Check sheet for the modelled part. Datum: model origin and axes. Units: mm. A direction names the side the tool comes from. Give positions to 0.01 mm unless a question says otherwise; leave off trailing zeros. Loops run counter-clockwise (first coordinate to the right, second up) from the corner with the lowest first, then second, coordinate; pieces in that order, holes last. Notation, with made-up numbers: (-10, -40) -> (18, -40) arc R19 ccw to (18, -24) -> close; hole circle Ø9 at (51, 1). An arc over 180 degrees is marked (long way). Write each question's results on one line, items separated by ' | '. Start each with the question number.
1. Cross-section at B-B on y = 12. Record the boundary of the cut face in (x, z), and give its area (3 significant figures).
2. Tool access check on faces 5 (the face through (-18.706, 25.35, -19.72)), 6 (the face through (-96, -1, 12)), 7 (the face through (-79, 31, 0)). Record the directions out of +Z, -Z, +X, -X, +Y, -Y that give a thin tool (end or side, any length) a straight path to the whole face; none if there is none.
3. Cross-section at C-C on z = -28. Record the boundary of the cut face in (x, y).
4. Mould release check, pull along Y, two halves, no side actions. Record for faces 1 (the face through (69.076, 6.007, 9.86)), 2 (the face through (-1, 50, 10)), 3 (the face through (-1, -46, 12)), 4 (the face through (26, 1, 0)): +Y half, -Y half, draft (parallel to the pull), parting line (faces both ways), or undercut.
5. Cross-section at A-A on x = 50. Record the boundary of the cut face in (y, z), and give its area (3 significant figures).
6. Gauge pin test, flat ends, axial feed: pin 1 Ø10 at (x, y) = (31, -2.5) entering from -Z; pin 2 Ø3 at (y, z) = (14.5, -11) entering from +X; pin 3 Ø4 at (x, z) = (-70.5, -9.5) entering from -Y. Record the tip position at first contact, or that the pin passes through.
7. Cross-section at D-D on x = 18.5. Record the boundary of the cut face in (y, z).
8. Material ranges on L1, parallel to Y at x = 50, z = 6; L2, parallel to Y at x = -11, z = 14; L3, parallel to Z at x = 9.5, y = 24, recorded low to high. Write a range as from..to.
from build123d import *

# Parameters (mm, degrees)
SKICA1_W                = 200
SKICA1_H                = 100
SKICA1_R                = 20
P_IDAT_VYSUNUT_M1_DEPTH = 20
ZAOBLIT1_R              = 10
SKO_EPINA1_T            = -4
P_IDAT_VYSUNUT_M2_DEPTH = 40


with BuildPart() as part:
    # Skica1 → Přidat vysunutím1 (new body)
    with BuildSketch(Plane.XY):
        Rectangle(SKICA1_W, SKICA1_H)
        with Locations((50, 0)):
            Circle(SKICA1_R, mode=Mode.SUBTRACT)
    extrude(amount=P_IDAT_VYSUNUT_M1_DEPTH)

    # Zaoblit1
    zaoblit1_edges = [part.edges().sort_by_distance(p)[0] for p in [
        (-100, 50, 10),
        (100, 50, 10),
        (100, -50, 10),
        (-100, -50, 10),
    ]]
    fillet(zaoblit1_edges, radius=ZAOBLIT1_R)

    # Skořepina1
    sko_epina1_openings = [part.faces().sort_by_distance(p)[0] for p in [
        (0, 0, 20),
    ]]
    offset(amount=SKO_EPINA1_T, openings=sko_epina1_openings, kind=Kind.INTERSECTION)

    # Skica2 → Přidat vysunutím2 (add)
    with BuildSketch(Plane(origin=(0, 0, 0), x_dir=(-1, 0, 0), z_dir=(0, 0, -1))):
        Polygon((45.55, -50), (100, 0), (45.55, 50), (-8.9, 0), align=None)
    extrude(amount=P_IDAT_VYSUNUT_M2_DEPTH)


solid = part.part
Geometry says:
1) outline: (-100, 0) -> (-86.93, 0) -> (-86.93, -40) -> (-4.17, -40) -> (-4.17, 0) -> (34, 0) -> (34, 20) -> (29.22, 20) -> (29.22, 4) -> (-96, 4) -> (-96, 20) -> (-100, 20) -> close; (66, 0) -> (100, 0) -> (100, 20) -> (96, 20) -> (96, 4) -> (70.78, 4) -> (70.78, 20) -> (66, 20) -> close | area: 4,260 mm^2
2) face 5: -Z, +X, +Y | face 6: +Z | face 7: -Z, -X, +Y
3) outline: (-100, 0) -> (-45.55, -50) -> (8.9, 0) -> (-45.55, 50) -> close
4) face 1: undercut | face 2: +Y half | face 3: undercut | face 4: draft
5) outline: (-50, 0) -> (-20, 0) -> (-20, 20) -> (-24, 20) -> (-24, 4) -> (-46, 4) -> (-46, 20) -> (-50, 20) -> close; (20, 0) -> (50, 0) -> (50, 20) -> (46, 20) -> (46, 4) -> (24, 4) -> (24, 20) -> (20, 20) -> close | area: 496 mm^2
6) pin 1: z = 0 | pin 2: x = -5.26 | pin 3: y = -28.93
7) outline: (-50, 0) -> (50, 0) -> (50, 20) -> (46, 20) -> (46, 4) -> (-46, 4) -> (-46, 20) -> (-50, 20) -> close
8) L1: -50..-46, -24..-20, 20..24, 46..50 | L2: -50..-46, 46..50 | L3: 0..4
